```python
from build123d import *

# Parameters (mm, degrees)
SKETCH1_R           = 1.5
BOSS_EXTRUDE1_DEPTH = 3


with BuildPart() as part:
    # Sketch1 → Boss-Extrude1 (new body)
    with BuildSketch(Plane(origin=(0, 0, 0), x_dir=(1, 0, 0), z_dir=(0, 1, 0))):
        with BuildLine():
            Line((15, 5), (15, -5))
            ThreePointArc((15, -5), (11.817238575, -8.915625252), (7.333939444, -6.6))
            ThreePointArc((7.333939444, -6.6), (6.965146863, -6.163339973), (6.417424305, -6))
            Line((6.417424305, -6), (-3, -6))
            ThreePointArc((-3, -6), (-4.414213562, -5.414213562), (-5, -4))
            Line((-5, -4), (-5, 4))
            ThreePointArc((-5, 4), (-4.414213562, 5.414213562), (-3, 6))
            Line((-3, 6), (6.417424305, 6))
            ThreePointArc((6.417424305, 6), (6.965146863, 6.163339973), (7.333939444, 6.6))
            ThreePointArc((7.333939444, 6.6), (11.817238575, 8.915625252), (15, 5))
        make_face()
        Circle(SKETCH1_R, mode=Mode.SUBTRACT)
        with Locations((11, 5)):
            Circle(SKETCH1_R, mode=Mode.SUBTRACT)
        with Locations((11, -5)):
            Circle(SKETCH1_R, mode=Mode.SUBTRACT)
    extrude(amount=BOSS_EXTRUDE1_DEPTH)


solid = part.part
```
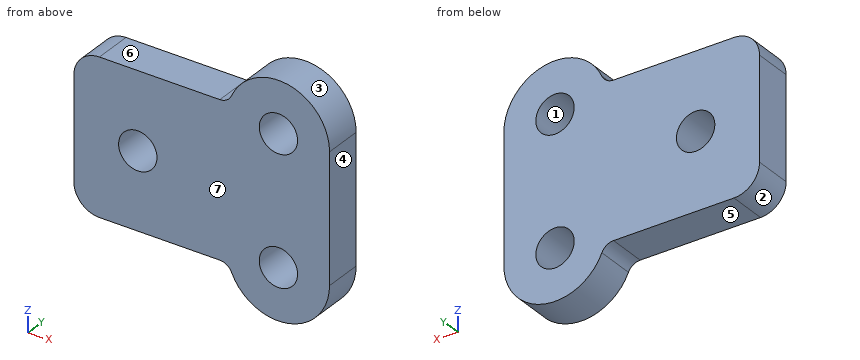
Could you check a few things on this model? Use its own coordinates, in mm. Face numbers are marked on the shaded views. A direction names the side the tool comes from. Round coordinates to 2 decimals unless told otherwise and drop trailing zeros. Loops run counter-clockwise (first coordinate to the right, second up) from the corner with the lowest first, then second, coordinate; pieces in that order, holes last. Notation, with made-up numbers: M -23.5,74.25 L -19.5,74.25 A15 ccw -19.5,85.25 Z; hole C 0.5,14 d4. An arc over 180 degrees is marked long. Put each result on its own line as item: value.
Q1. Imagine slicing it at D-D (x = 0). Write out the boundary of the cut face in (y, z), then the cut area to 3 significant figures.
Check result:
outline: M 0,-6 L 3,-6 L 3,-1.5 L 0,-1.5 Z; M 0,1.5 L 3,1.5 L 3,6 L 0,6 Z
area: 27.0 mm2
Q2. Thinking about a two-plate mould opening in Z: for the marked faces 1, 2, 3 and 4, which applies, released by +Z, released by -Z, zero draft, split by the parting line, or undercut?
Check result:
face 1: undercut
face 2: released by -Z
face 3: released by +Z
face 4: zero draft
Q3. Imagine slicing it at C-C (y = 2.2). Write out the boundary of the cut face in (x, z), then the cut area to 3 significant figures.
Check result:
outline: M -5,-4 A2 ccw -3,-6 L 6.42,-6 A1 cw 7.33,-6.6 A4 ccw 15,-5 L 15,5 A4 ccw 7.33,6.6 A1 cw 6.42,6 L -3,6 A2 ccw -5,4 Z; hole C 0,0 d3; hole C 11,-5 d3; hole C 11,5 d3
area: 252 mm2
Q4. Imagine slicing it at B-B (x = 11). Write out the boundary of the cut face in (y, z), then the cut area to 3 significant figures.
Check result:
outline: M 0,-9 L 3,-9 L 3,-6.5 L 0,-6.5 Z; M 0,-3.5 L 3,-3.5 L 3,3.5 L 0,3.5 Z; M 0,6.5 L 3,6.5 L 3,9 L 0,9 Z
area: 36.0 mm2
Q5. I need wall thicknesses on probe 1 along Z at (x, y) = (11, 1.55); probe 2 along Z at (x, y) = (0, 2.2); probe 3 along X at (y, z) = (2, 0). Which ranges of each line are inside material? Lowest first, please.
Check result:
probe 1: -9 to -6.5, -3.5 to 3.5, 6.5 to 9
probe 2: -6 to -1.5, 1.5 to 6
probe 3: -5 to -1.5, 1.5 to 15
Q6. On a 3-axis mill with a long thin cutter (end or side, diameter ignored), from which of +Z, -Z, +X, -X, +Y, -Y can I reach the whole of each face in a straight line? I mean the marked faces 5, 6 and 7. Say none if no direction works.
Check result:
face 5: -Z, -X, +Y, -Y
face 6: +Z, -X, +Y, -Y
face 7: +Z, -Z, +X, -X, -Y
Q7. Imagine slicing it at A-A (z = 0). Write out the boundary of the cut face in (x, y), then the cut area to 3 significant figures.
Check result:
outline: M -5,0 L -1.5,0 L -1.5,3 L -5,3 Z; M 1.5,0 L 15,0 L 15,3 L 1.5,3 Z
area: 51.0 mm2
Q8. For pin 1 (1.5 mm diameter, centred on x = 0, y = 1.5, fed in from -Z), with a flat end and sliding along its axis, tell me the tip position at first contact or that it passes through.
Check result:
pin 1: z = -6
